Read the model definition and answer for the solid it produces. Units are mm, in the model's axes. Face numbers are marked on the shaded views. A direction names the side the tool comes from. Coordinates: 2 decimals unless noted, no trailing zeros. Order: outer loops, then holes, each group sorted by start corner. A loop starts at its lowest first (then second) coordinate and runs counter-clockwise, first axis right, second up. Notation, with made-up numbers: M -19,48 L 35,48 A30 ccw 35,85 Z; hole C 1.25,-13.5 d11. An arc over 180 degrees is marked long. Write each question's results on one line, items separated by ' | '.
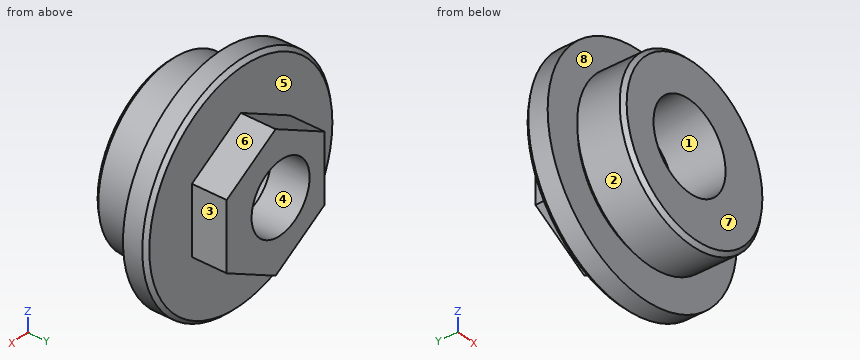
Autodesk Inventor part; units mm, degrees
ref_plane "YZ Plane" through (0, 0, 0) normal (1, 0, 0) x (0, 1, 0)
ref_plane "XZ Plane" through (0, 0, 0) normal (0, 1, 0) x (-1, 0, 0)
ref_plane "XY Plane" through (0, 0, 0) normal (0, 0, 1) x (1, 0, 0)
sketch "草图1" plane through (0, 0, 0) normal (0, 1, 0) x (-1, 0, 0)
  circle A0 centre (0, 0) radius 60
  dimension "d0" = 120
extrude "拉伸1" add sketch "草图1" along normal mid plane 12
sketch "草图2" plane through (0, -6, 0) normal (0, -1, 0) x (1, 0, 0)
  circle A0 centre (0, 0) radius 41
  dimension "d3" = 82
extrude "拉伸2" add sketch "草图2" along normal blind 3
sketch "草图3" plane through (0, -9, 0) normal (0, -1, 0) x (1, 0, 0)
  circle A0 centre (0, 0) radius 45
  dimension "d6" = 90
extrude "拉伸3" add sketch "草图3" along normal blind 24
thread "螺纹1"
sketch "草图4" plane through (0, 6, 0) normal (0, 1, 0) x (1, 0, 0)
  line L0 (-31, 17.8979) -> (0, 35.7957)
  line L1 (0, 35.7957) -> (31, 17.8979)
  line L2 (31, 17.8979) -> (31, -17.8979)
  line L3 (31, -17.8979) -> (0, -35.7957)
  line L4 (0, -35.7957) -> (-31, -17.8979)
  line L5 (-31, -17.8979) -> (-31, 17.8979)
  point P0 (0, 0)
  point P1 (0, 0)
  dimension "d11" = 62
extrude "拉伸4" add sketch "草图4" along normal blind 18
sketch "草图5" plane through (0, 24, 0) normal (0, 1, 0) x (1, 0, 0)
  line L0 (0, 35.7957) -> (-31, 17.8979)
  point P0 (0, 0)
  point P1 (-3.1488, -0.6537)
  dimension "d14" = 29.9917
hole "孔1" at (-3.1488, 24, 0.6537) direction (0, -1, 0) diameter 36.7524 depth 20
sketch "草图6" plane through (-3.1488, 4, 0.6537) normal (0, 1, 0) x (1, 0, 0)
  circle A0 centre (0, 0) radius 18.3762
  point P0 (3.1488, 0.6537)
hole "孔2" at (-3.1488, 4, 0.6537) direction (0, -1, 0) diameter 41 depth 5
sketch "草图7" plane through (-3.1488, -1, 0.6537) normal (0, 1, 0) x (1, 0, 0)
  circle A0 centre (0, 0) radius 20.5
  point P0 (3.1488, 0.6537)
hole "孔3" at (-3.1488, -1, 0.6537) direction (0, -1, 0) diameter 22 depth 5
sketch "草图8" plane through (-3.1488, -6, 0.6537) normal (0, 1, 0) x (1, 0, 0)
  circle A0 centre (0, 0) radius 11
  point P0 (3.1488, 0.6537)
hole "孔4" at (-3.1488, -6, 0.6537) direction (0, -1, 0) diameter 45.6699 end through all
chamfer "倒角1" distance 2 angle 45 2 edges at (60, 6, 0) (-45, -33, 0)
properties part number "螺盖" material "不锈钢"
(1) The part is cut by section B-B, the plane y = -23. Write down the section's boundary in (x, z).
Conclusion:
outline: C 0,0 d90; hole C -3.15,0.65 d45.67
(2) For the marked faces 5, 6, 7 and 8, determine the directions among +Z, -Z, +X, -X, +Y, -Y from which every point of the face is accessible in a straight line to the end or side of a thin tool.
Conclusion:
face 5: +Y | face 6: +Z, +X, +Y | face 7: +Z, -Z, +X, -X, -Y | face 8: none
(3) The part is cut by section A-A, the plane y = 9.5. Write down the section's boundary in (x, z), then the cut area to 3 significant figures.
Conclusion:
outline: M -31,-17.9 L 0,-35.8 L 31,-17.9 L 31,17.9 L 0,35.8 L -31,17.9 Z; hole C -3.15,0.65 d36.75 | area: 2,270 mm²
(4) Straight lines are drawn through the part: line 1 (Y direction, x = 31.5, z = -8); line 2 (Z direction, x = 7, y = -13); line 3 (Z direction, x = -4.5, y = 5.5). For each, find the intervals that lie inside material, in ascending order.
Conclusion:
line 1: -33 to 6 | line 2: -44.45 to -19.8, 21.11 to 44.45 | line 3: -58.33 to -17.67, 18.98 to 58.33
(5) The mould has two halves that part along X. Classify the marked faces 1, 2, 3 and 4: pulls with the +X half, pulls with the -X half, needs draft (parallel to the pull), parting line crosses it, or undercut.
Conclusion:
face 1: undercut | face 2: parting line crosses it | face 3: pulls with the +X half | face 4: undercut
(6) Given pin 1 (10 mm diameter, centred on y = 9, z = 20, fed in from +X); pin 2 (5.5 mm diameter, centred on y = 17, z = -6.5, fed in from -X); pin 3 (12.5 mm diameter, centred on x = -10, z = 9.5, fed in from +Y); pin 4 (20 mm diameter, centred on x = -3.15, z = 0.65, fed in from +Y), each flat-ended and moving along its own axis, determine where each tip first touches the part or whether it passes through.
Conclusion:
pin 1: x = 56.83 | pin 2: x = -31 | pin 3: y = -1 | pin 4: through
